Check sheet for the drawn part. Datum: minimum x, y, z corner. Units: mm. A direction names the side the tool comes from. Coordinates: 2 decimals unless noted, no trailing zeros. Order: outer loops, then holes, each group sorted by start corner. A loop starts at its lowest first (then second) coordinate and runs counter-clockwise, first axis right, second up. Notation, with made-up numbers: (87.25, 5.5) - (95.25, 5.5) arc R13 ccw to (95.25, 27.5) - close; hole circle Ø8 at (72, 18.5). An arc over 180 degrees is marked (long way). Return JSON: item names as keys, results as strings. Group by question number.
Item 1: Scan lines: probe 1 along X at (y, z) = (30.6, 34.6); probe 2 along Y at (x, z) = (30, 33). Record each from-to range of solid material in increasing order.
Item 2: Gauge pin test, flat ends, axial feed: pin 1 (1.5 mm diameter, centred on x = 7, y = 29.5, fed in from +Z); pin 2 (1.5 mm diameter, centred on x = 26, y = 12, fed in from +Z); pin 3 (2 mm diameter, centred on x = 4.6, y = 4.6, fed in from +Z); pin 4 (4 mm diameter, centred on x = 30.6, y = 30.6, fed in from -Z). Record the tip position at first contact, or that the pin passes through.
Item 3: Tool access check on the marked faces 1 and 2. Record the directions out of +Z, -Z, +X, -X, +Y, -Y that give a thin tool (end or side, any length) a straight path to the whole face; none if there is none.
Item 4: Section check A-A on z = 5.5. Enter the section's corners in (x, y).
Item 5: Section check D-D on z = 46. Enter the section's corners in (x, y).
Item 6: Section check B-B on y = 17.6. Enter the section's corners in (x, z).
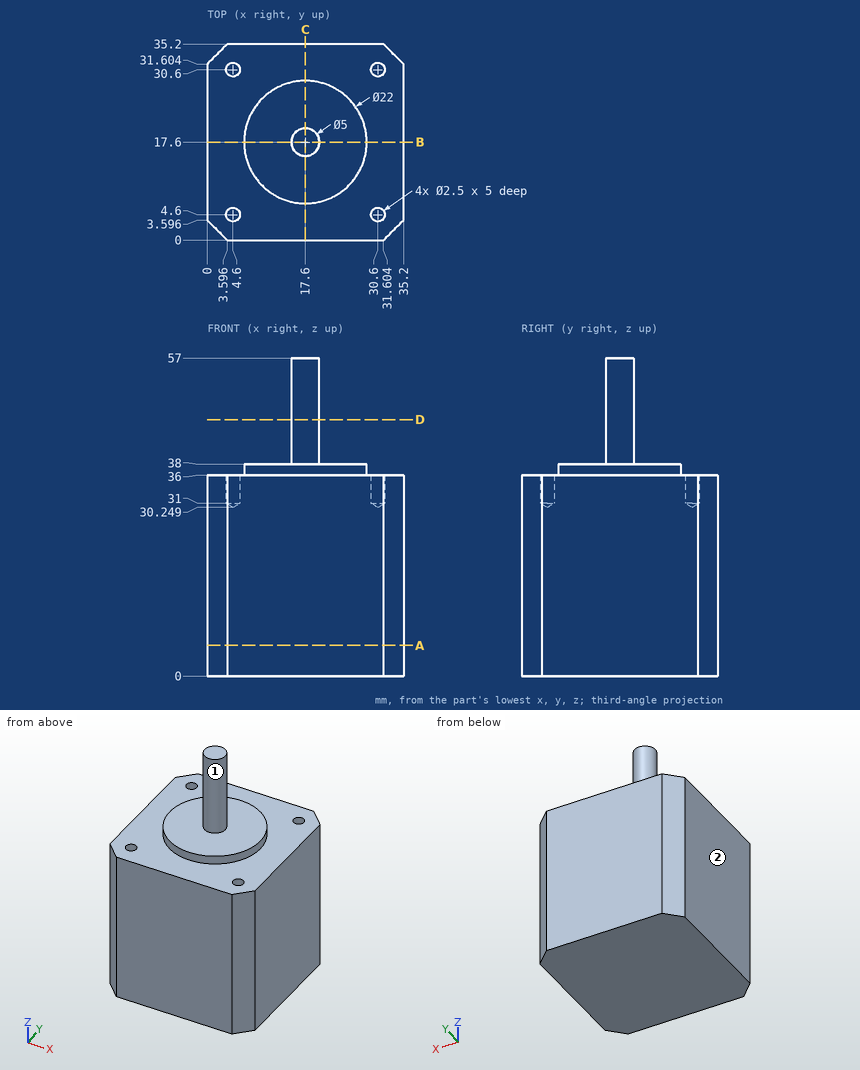
Computed:
{
 "1": {"probe 1": "x = 0 to 3.35, 5.85 to 29.35, 31.85 to 35.2", "probe 2": "y = 0 to 3.5, 5.7 to 29.5, 31.7 to 35.2"},
 "2": {"pin 1": "stops at z = 36", "pin 2": "stops at z = 38", "pin 3": "stops at z = 30.85", "pin 4": "stops at z = 0"},
 "3": {"face 1": "+Z", "face 2": "+Z, -Z, -X, +Y, -Y"},
 "4": {"outline": "(0, 3.6) - (3.6, 0) - (31.6, 0) - (35.2, 3.6) - (35.2, 31.6) - (31.6, 35.2) - (3.6, 35.2) - (0, 31.6) - close"},
 "5": {"outline": "circle Ø5 at (17.6, 17.6)"},
 "6": {"outline": "(0, 0) - (35.2, 0) - (35.2, 36) - (28.6, 36) - (28.6, 38) - (20.1, 38) - (20.1, 57) - (15.1, 57) - (15.1, 38) - (6.6, 38) - (6.6, 36) - (0, 36) - close"}
}
